The figure shows three views and two pictorial views of one solid part (mm, origin at its lowest corner). Answer the questions. Coordinates: 2 decimals unless noted, no trailing zeros. Order: outer loops, then holes, each group sorted by start corner. A loop starts at its lowest first (then second) coordinate and runs counter-clockwise, first axis right, second up. Notation, with made-up numbers: M -6,-1 L 21,-1 A31 ccw 21,30 Z; hole C 10,-36 d7. An arc over 180 degrees is marked long. Answer in a Markdown table with one row per item. Add a question column.
Item 1: Consider line 1 (Y direction, x = 7.75, z = 12.5) (1 decimal); line 2 (X direction, y = 8, z = 11.75); line 3 (Z direction, x = 7, y = 20) (1 decimal). Determine where each line is inside the solid, lowest interval first. Write a range as from..to.
Item 2: The part is cut by section B-B (y = 9.5). Write down the section's boundary in (x, z).
Item 3: The part is cut by section A-A (x = 15.75). Write down the section's boundary in (y, z).
Item 4: The part is cut by section D-D (x = 8.75). Write down the section's boundary in (y, z) (1 decimal).
Item 5: The mould has two halves that part along Z. Classify the marked faces 1, 2, 3 and 4: released by +Z, released by -Z, zero draft, split by the parting line, or undercut.
Item 6: The part is cut by section C-C (z = 21.75). Write down the section's boundary in (x, y), then the cut area to 3 significant figures.
Item 7: Flat-ended cylindrical pins translate along their axes: pin 1 Ø11 at (y, z) = (17, 14) entering from -X; pin 2 Ø3 at (x, y) = (2.5, 4) entering from +Z (1 decimal); pin 3 Ø5 at (x, z) = (2, 5) entering from -Y. Find the tip coordinate at first contact, or state that the pin passes through.
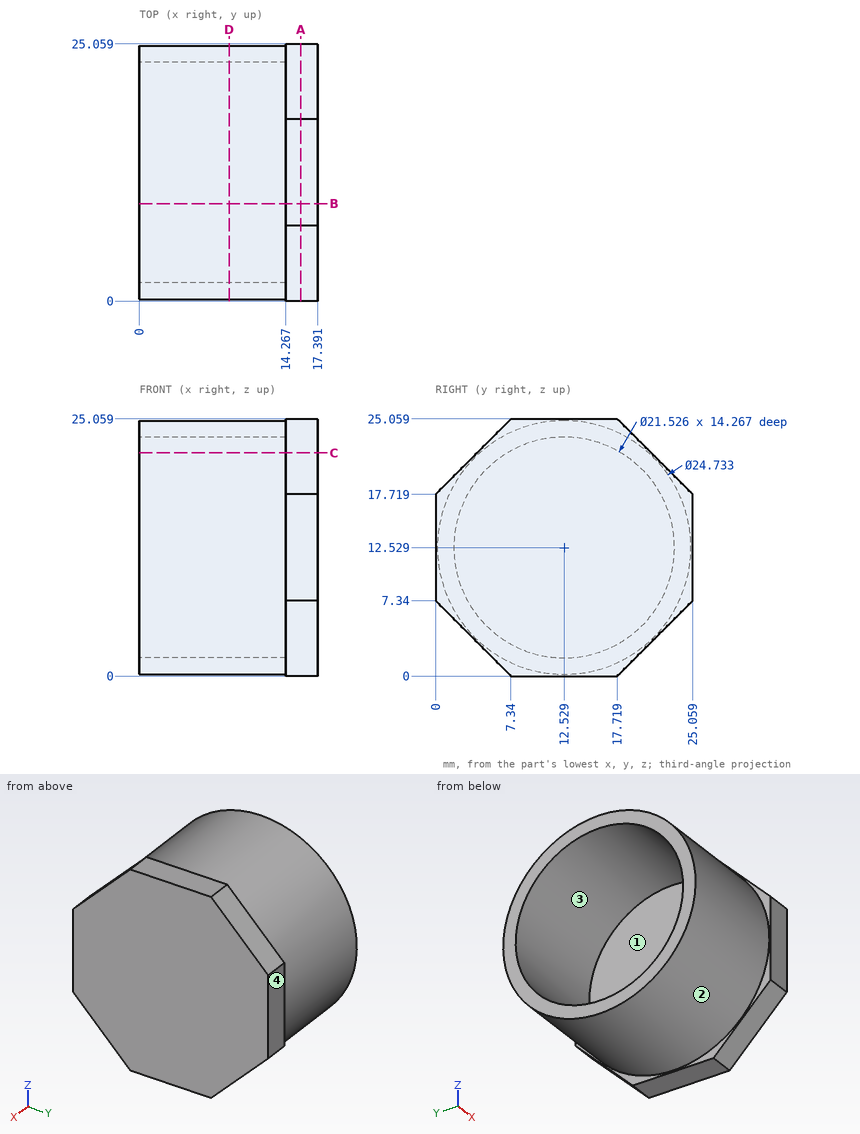
Reply:
| question | item | result |
|---|---|---|
| 1 | line 1 | y = 0.2..1.8, 23.3..24.9 |
| 1 | line 2 | x = 14.27..17.39 |
| 1 | line 3 | z = 2.7..4.8, 20.3..22.4 |
| 2 | outline | M 0,0.54 L 14.27,0.54 L 14.27,0 L 17.39,0 L 17.39,25.06 L 14.27,25.06 L 14.27,24.52 L 0,24.52 L 0,22.86 L 14.27,22.86 L 14.27,2.2 L 0,2.2 Z |
| 3 | outline | M 0,7.34 L 7.34,0 L 17.72,0 L 25.06,7.34 L 25.06,17.72 L 17.72,25.06 L 7.34,25.06 L 0,17.72 Z |
| 4 | outline | C 12.5,12.5 d24.7; hole C 12.5,12.5 d21.5 |
| 5 | face 1 | undercut |
| 5 | face 2 | split by the parting line |
| 5 | face 3 | undercut |
| 5 | face 4 | zero draft |
| 6 | outline | M 0,4.29 L 14.27,4.29 L 14.27,4.03 L 17.39,4.03 L 17.39,21.03 L 14.27,21.03 L 14.27,20.77 L 0,20.77 L 0,18.08 L 14.27,18.08 L 14.27,6.98 L 0,6.98 Z |
| 6 | area | 130 mm2 |
| 7 | pin 1 | stops at x = 14.27 |
| 7 | pin 2 | stops at z = 22.7 |
| 7 | pin 3 | stops at y = 1.23 |
